```python
from build123d import *
from build123d.topology import SkipClean

# Parameters (mm, degrees)
SCHIZZO1_R                    = 4
ESTRUSIONE_ESTRUSIONE1_DEPTH  = 40.625
SCHIZZO3_R                    = 4
TAGLIO_ESTRUSIONE1_START      = 40.625
TAGLIO_ESTRUSIONE1_DEPTH      = 1.1
TAGLIO_ESTRUSIONE2_START      = -39.625
TAGLIO_ESTRUSIONE2_DEPTH      = 1
TAGLIO_ESTRUSIONE3_START      = -40.625
SCHIZZO6_R                    = 1.5
TAGLIO_ESTRUSIONE3_DEPTH      = 6
TAGLIO_ESTRUSIONE4_START      = 34.625
SCHIZZO7_R                    = 1.5
TAGLIO_ESTRUSIONE4_DEPTH      = 6
TAGLIO_ESTRUSIONE5_START      = 5
TAGLIO_ESTRUSIONE5_DEPTH      = 6
TAGLIO_ESTRUSIONE7_DEPTH      = 56.95924295
TAGLIO_ESTRUSIONE7_DEPTH_BACK = 56.95924295
SCHIZZO9_W                    = 63.05
SCHIZZO9_H                    = 4.127016654


with BuildPart() as part:
    # Schizzo1 → Estrusione-Estrusione1 (new, symmetric)
    with BuildSketch(Plane(origin=(0, 0, 0), x_dir=(0, 0, -1), z_dir=(1, 0, 0))):
        Circle(SCHIZZO1_R)
    extrude(amount=ESTRUSIONE_ESTRUSIONE1_DEPTH, both=True)

    # Sweep1: sweep along a path in Schizzo2
    with BuildLine(Plane.XY) as sweep1_path:
        Line((-20.625, 0), (-14.503941276, 23.206306042))
        ThreePointArc((-14.503941276, 23.206306042), (0, 34.380644339), (14.503941276, 23.206306042))
        Line((14.503941276, 23.206306042), (20.625, 0))
    # Schizzo3 → Sweep1 (sweep)
    with BuildSketch(Plane(origin=(0, 0, 0), x_dir=(1, 0, 0), z_dir=(0, 1, 0))):
        with Locations((-20.625, 0)):
            Circle(SCHIZZO3_R)
    sweep(path=sweep1_path.line)

    # Schizzo4 → Taglio-Estrusione1 (cut)
    with BuildSketch(Plane(origin=(0, 0, 0), x_dir=(0, 0, -1), z_dir=(1, 0, 0)).offset(TAGLIO_ESTRUSIONE1_START)):
        with BuildLine():
            ThreePointArc((-0.009903808, -2.999983652), (0.509762562, 2.956373138), (-0.995361521, -2.830062798))
            Line((-0.995361521, -2.830062798), (-1.16, -3.828106582))
            ThreePointArc((-1.16, -3.828106582), (0.672388498, 3.943081753), (-0.174229562, -3.996203706))
            Line((-0.174229562, -3.996203706), (-0.009903808, -2.999983652))
        make_face()
    extrude(amount=-TAGLIO_ESTRUSIONE1_DEPTH, mode=Mode.SUBTRACT)

    # Schizzo5 → Taglio-Estrusione2 (cut)
    with BuildSketch(Plane(origin=(0, 0, 0), x_dir=(0, 0, -1), z_dir=(1, 0, 0)).offset(TAGLIO_ESTRUSIONE2_START)):
        with BuildLine():
            Line((-1.16, -3.828106582), (-0.995361521, -2.830062798))
            ThreePointArc((-0.995361521, -2.830062798), (0.509762562, 2.956373138), (-0.009903808, -2.999983652))
            Line((-0.009903808, -2.999983652), (-0.174229562, -3.996203706))
            ThreePointArc((-0.174229562, -3.996203706), (0.672388498, 3.943081753), (-1.16, -3.828106582))
        make_face()
    extrude(amount=-TAGLIO_ESTRUSIONE2_DEPTH, mode=Mode.SUBTRACT)

    # Schizzo6 → Taglio-Estrusione3 (cut)
    with BuildSketch(Plane(origin=(0, 0, 0), x_dir=(0, 0, -1), z_dir=(1, 0, 0)).offset(TAGLIO_ESTRUSIONE3_START)):
        Circle(SCHIZZO6_R)
    extrude(amount=TAGLIO_ESTRUSIONE3_DEPTH, mode=Mode.SUBTRACT)

    # Schizzo7 → Taglio-Estrusione4 (cut)
    with BuildSketch(Plane(origin=(0, 0, 0), x_dir=(0, 0, -1), z_dir=(1, 0, 0)).offset(TAGLIO_ESTRUSIONE4_START)):
        Circle(SCHIZZO7_R)
    extrude(amount=TAGLIO_ESTRUSIONE4_DEPTH, mode=Mode.SUBTRACT)

    # Schizzo8 → Taglio-Estrusione5 (cut)
    with SkipClean():  # the faces are left unmerged after this step: merging them gives an invalid solid
        with BuildSketch(Plane.XY.offset(TAGLIO_ESTRUSIONE5_START)):
            with BuildLine():
                Line((-31.525, -3.5), (31.525, -3.5))
                Line((31.525, -3.5), (31.525, 3.5))
                Line((31.525, 3.5), (23.184714524, 3.5))
                Line((23.184714524, 3.5), (23.086467119, 3.872477943))
                Line((23.086467119, 3.872477943), (17.503564721, 25.038512689))
                ThreePointArc((17.503564721, 25.038512689), (-1.006578206, 37.748362013), (-18.017008414, 23.091932531))
                Line((-18.017008414, 23.091932531), (-23.086467119, 3.872477943))
                Line((-23.086467119, 3.872477943), (-23.184714524, 3.5))
                Line((-23.184714524, 3.5), (-31.525, 3.5))
                Line((-31.525, 3.5), (-31.525, -3.5))
            make_face()
            with BuildLine():
                Line((-16.053396537, 4.127522057), (-10.981638972, 23.355692138))
                ThreePointArc((-10.981638972, 23.355692138), (1.042788279, 31.012926666), (11.513552997, 21.339086809))
                Line((11.513552997, 21.339086809), (16.053396537, 4.127522057))
                Line((16.053396537, 4.127522057), (16.218916174, 3.5))
                Line((16.218916174, 3.5), (-16.218916174, 3.5))
                Line((-16.218916174, 3.5), (-16.053396537, 4.127522057))
            make_face(mode=Mode.SUBTRACT)
        extrude(amount=-TAGLIO_ESTRUSIONE5_DEPTH, mode=Mode.SUBTRACT)

    # Schizzo9 → Taglio-Estrusione7 (cut, two sides: drawn at the far end of the back side and taken through both)
    with BuildSketch(Plane(origin=(0, 0, 0), x_dir=(1, 0, 0), z_dir=(0, 1, 0)).offset(-TAGLIO_ESTRUSIONE7_DEPTH_BACK)):
        with Locations((0, -1.936491673)):
            Rectangle(SCHIZZO9_W, SCHIZZO9_H)
    extrude(amount=TAGLIO_ESTRUSIONE7_DEPTH + TAGLIO_ESTRUSIONE7_DEPTH_BACK, mode=Mode.SUBTRACT)


solid = part.part
```
Check sheet for the modelled part. Datum: model origin and axes. Units: mm. A direction names the side the tool comes from. Give positions to 0.01 mm unless a question says otherwise; leave off trailing zeros. Write each loop counter-clockwise with the first axis right and the second up, starting at its lowest first coordinate (ties: lowest second). Pieces come first, ordered by that corner, then holes. Notation, with made-up numbers: (70.25, 10) - (123.25, 10) arc R18 ccw to (123.25, 28) - close; hole circle Ø7 at (49.5, -37.75). An arc over 180 degrees is marked (long way). Answer as a JSON object with one key per item and string values. Group by question number.
1) Access from +Z, -Z, +X, -X, +Y, -Y to the whole of each face (thin tool, end or side, straight path). Record for faces 1 (the face through (39.525, -3, -1)), 2 (the face through (0.569, -1.532, -3.695)), 3 (the face through (31.525, 0, 1)), 4 (the face through (-40, 3, 0)).
2) Sectioned sample at A-A (x = -33.5). Record the cut outline in (y, z).
3) Release check for a two-part mould opening along Z. For faces 5 (the face through (40.083, 2.933, -0.632)), 6 (the face through (-39.625, -3, -1)), 7 (the face through (-11.8, 33.7, -0.127)), 8 (the face through (37.58, 0.07, 1.5)) record: pulls with the +Z half, pulls with the -Z half, needs draft (parallel to the pull), parting line crosses it, or undercut.
4) Thickness scan on probe 1 along Y at (x, z) = (36.65, 0); probe 2 along X at (y, z) = (8, -0.5); probe 3 along X at (y, z) = (18, -2.75). Record the ranges inside material, lowest first. Write a range as from..to.
5) Depth check by flat-ended pin: P1, Ø2.5, axis at y = 0, z = 0, coming from the -X side (3 decimals); P2, Ø1, axis at x = 26.5, z = -0.5, coming from the -Y side; P3, Ø8.5, axis at x = 4, y = 23, coming from the +Z side; P4, Ø17.5, axis at x = -5.5, y = 12.5, coming from the +Z side. Enter the tip coordinate at first touch or a pass-through.
Geometry results:
{
 "1": {"face 1": "+X", "face 2": "none", "face 3": "+Z", "face 4": "-X"},
 "2": {"outline": "circle Ø8 at (0, 0)"},
 "3": {"face 5": "parting line crosses it", "face 6": "needs draft", "face 7": "pulls with the +Z half", "face 8": "undercut"},
 "4": {"probe 1": "y = -4..-1.5, 1.5..4", "probe 2": "x = -22.48..-22, -15.03..-14.55, 14.55..15.03, 22..22.48", "probe 3": "x = -18.78..-12.97, 12.97..18.78"},
 "5": {"P1": "stops at x = -34.625", "P2": "stops at y = -4", "P3": "passes through", "P4": "stops at z = -0.13"}
}
